from build123d import *

# Parameters (mm, degrees)
BOSS_EXTRUDE1_DEPTH = 20
SKETCH1_2_W         = 21.5
SKETCH1_2_H         = 60
BOSS_EXTRUDE2_DEPTH = 50
SKETCH3_W           = 40
SKETCH3_H           = 50
CUT_EXTRUDE1_DEPTH  = 50
SKETCH4_R           = 2
CUT_EXTRUDE2_DEPTH  = 50


with BuildPart() as part:
    # Sketch1 → Boss-Extrude1 (new body)
    with BuildSketch(Plane.XY):
        Polygon((0, 8), (0, 50), (0, 110), (-21.5, 110), (-21.5, 50), (-21.5, 0), (0, 0), (0, 5), (-16.5, 5), (-16.5, 8), align=None)
    extrude(amount=BOSS_EXTRUDE1_DEPTH)

    # Sketch1_2 → Boss-Extrude2 (add)
    with BuildSketch(Plane.XY):
        with Locations((-10.75, 80)):
            Rectangle(SKETCH1_2_W, SKETCH1_2_H)
    extrude(amount=BOSS_EXTRUDE2_DEPTH)

    # Sketch3 → Cut-Extrude1 (cut)
    with BuildSketch(Plane(origin=(0, 0, 0), x_dir=(0, 0, -1), z_dir=(1, 0, 0))):
        with Locations((-20, 85)):
            Rectangle(SKETCH3_W, SKETCH3_H)
    extrude(amount=-CUT_EXTRUDE1_DEPTH, mode=Mode.SUBTRACT)

    # Sketch4 → Cut-Extrude2 (cut)
    with BuildSketch(Plane(origin=(0, 0, 40), x_dir=(-1, 0, 0), z_dir=(0, 0, -1))):
        with Locations(Location((10.75, 100, 0), (0, 0, 90))):
            Circle(SKETCH4_R)
    extrude(amount=-CUT_EXTRUDE2_DEPTH, mode=Mode.SUBTRACT)


solid = part.part
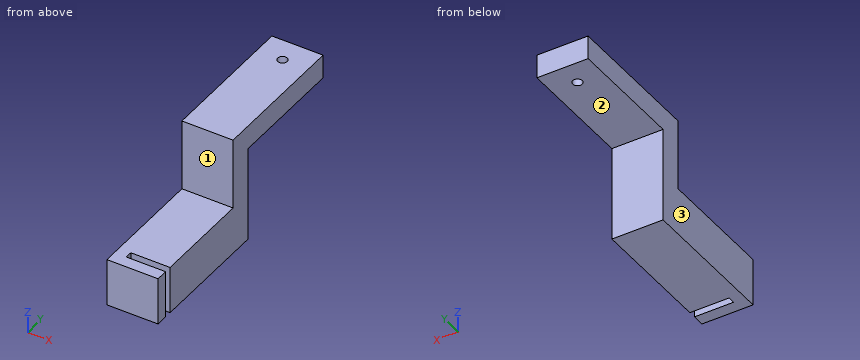
Geometry check sheet. Reference: the model listing, model coordinates, mm. Face numbers are marked on the shaded views. A direction names the side the tool comes from. Coordinates: 2 decimals unless noted, no trailing zeros. Loops run counter-clockwise (first coordinate to the right, second up) from the corner with the lowest first, then second, coordinate; pieces in that order, holes last. Notation, with made-up numbers: (77.25, -39.75) - (130.25, -39.75) arc R17 ccw to (130.25, -18.75) - close; hole circle Ø8 at (-16, 38). An arc over 180 degrees is marked (long way). Use one line per item in the form item = value. Start each with the question number.
Item 1: Thickness scan on probe 1 along X at (y, z) = (100, 42); probe 2 along Y at (x, z) = (-15.5, 14); probe 3 along Z at (x, y) = (-10.5, 96). Record the ranges inside material, lowest first.
Item 2: Section check C-C, the plane x = -10.75. Enter the section's corners in (y, z), and give its area (3 significant figures).
Item 3: Tool access check on the marked faces 1, 2 and 3. Record the directions out of +Z, -Z, +X, -X, +Y, -Y that give a thin tool (end or side, any length) a straight path to the whole face; none if there is none.
Item 4: Section check A-A, the plane x = -4.5. Enter the section's corners in (y, z).
Item 5: Section check D-D, the plane z = 19. Enter the section's corners in (x, y).
Item 6: Gauge pin test, flat ends, axial feed: pin 1 (1.5 mm diameter, centred on x = -14, z = 13, fed in from +Y); pin 2 (6 mm diameter, centred on x = -16.5, y = 66, fed in from -Z). Record the tip position at first contact, or that the pin passes through.
Item 7: Section check B-B, the plane y = 100. Enter the section's corners in (x, z).
Computed:
q1.probe_1 = -21.5 to -12.75, -8.75 to 0
q1.probe_2 = 0 to 5, 8 to 60
q1.probe_3 = 40 to 50
q2.outline = (0, 0) - (5, 0) - (5, 20) - (0, 20) - close; (8, 0) - (60, 0) - (60, 40) - (98, 40) - (98, 50) - (50, 50) - (50, 20) - (8, 20) - close; (102, 40) - (110, 40) - (110, 50) - (102, 50) - close
q2.area = 1,900 mm2
q3.face_1 = +Z, +X, -X, -Y
q3.face_2 = -Z, +X, -X, +Y
q3.face_3 = +Z, -Z, -X, +Y, -Y
q4.outline = (0, 0) - (5, 0) - (5, 20) - (0, 20) - close; (8, 0) - (60, 0) - (60, 40) - (110, 40) - (110, 50) - (50, 50) - (50, 20) - (8, 20) - close
q5.outline = (-21.5, 0) - (0, 0) - (0, 5) - (-16.5, 5) - (-16.5, 8) - (0, 8) - (0, 60) - (-21.5, 60) - close
q6.pin_1 = 60
q6.pin_2 = 40
q7.outline = (-21.5, 40) - (-12.75, 40) - (-12.75, 50) - (-21.5, 50) - close; (-8.75, 40) - (0, 40) - (0, 50) - (-8.75, 50) - close
